from build123d import *

# Parameters (mm, degrees)
F3_DEPTH        = 4
F4_DEPTH        = 4
F7_D            = 3.2
F7_DEPTH        = 45
F7_TIP          = 0.9613769904
F8_D            = 28
F10_D           = 3.2
F10_DEPTH       = 60
F10_CSINK_D     = 6.72
F10_CSINK_ANGLE = 90
F10_TIP         = 0.9613769904
F12_DEPTH       = 4.0010001
F13_R           = 5


with BuildPart() as f3:
    # F0 (on Top) → F3 (new body)
    with BuildSketch(Plane.XY):
        with BuildLine():
            Line((-83.330666624, 34), (83.330666624, 34))
            ThreePointArc((83.330666624, 34), (73.1470337796, 52.4357840529), (58.9576118919, 68))
            Line((58.9576118919, 68), (-58.9576118919, 68))
            Line((-58.9576118919, 68), (-108.330666624, 68))
            Line((-108.330666624, 68), (-108.330666624, 34))
            Line((-108.330666624, 34), (-83.330666624, 34))
        make_face()
    extrude(amount=F3_DEPTH)

    # F0 (on Top) → F4 (join)
    with BuildSketch(Plane.XY):
        with BuildLine():
            Line((-83.330666624, 34), (83.330666624, 34))
            ThreePointArc((83.330666624, 34), (73.1470337796, 52.4357840529), (58.9576118919, 68))
            Line((58.9576118919, 68), (-58.9576118919, 68))
            Line((-58.9576118919, 68), (-108.330666624, 68))
            Line((-108.330666624, 68), (-108.330666624, 34))
            Line((-108.330666624, 34), (-83.330666624, 34))
        make_face()
    extrude(amount=F4_DEPTH)

    # F7
    with Locations(Plane.YZ.offset(83.3)):
        with Locations((63, 2), (39, 2)):
            Hole(F7_D / 2, depth=F7_DEPTH)
            with Locations((0, 0, -(F7_DEPTH + F7_TIP / 2))):  # 118° drill point
                Cone(0, F7_D / 2, F7_TIP, mode=Mode.SUBTRACT)

    # F8 (through all)
    with Locations(Plane(origin=(0, 0, 0), x_dir=(1, 0, 0), z_dir=(0, 0, -1))):
        with Locations((0, -52)):
            Hole(F8_D / 2)

    # F10
    with Locations(Plane.XY.offset(4)):
        with Locations((-103.330666624, 51), (-90.330666624, 51)):
            CounterSinkHole(F10_D / 2, F10_CSINK_D / 2, depth=F10_DEPTH, counter_sink_angle=F10_CSINK_ANGLE)
            with Locations((0, 0, -(F10_DEPTH + F10_TIP / 2))):  # 118° drill point
                Cone(0, F10_D / 2, F10_TIP, mode=Mode.SUBTRACT)

    # F11 (on face) → F12 (cut, through all)
    with BuildSketch(Plane.XY.offset(4)):
        with BuildLine():
            ThreePointArc((-81.8600177132, 38), (-73.8985762248, 51.8079427496), (-63.6322441848, 64))
            Line((-63.6322441848, 64), (-65.1300137514, 65.3254004397))
            ThreePointArc((-65.1300137514, 65.3254004397), (-75.5329519196, 52.9537515968), (-83.6166513022, 38.9561581637))
            Line((-83.6166513022, 38.9561581637), (-81.8600177132, 38))
        make_face()
    extrude(amount=-F12_DEPTH, mode=Mode.SUBTRACT)

    # F13
    f13_edges = [f3.edges().sort_by_distance(p)[0] for p in [
        (-108.330667, 34, 2),
        (-108.330667, 68, 2),
    ]]
    fillet(f13_edges, radius=F13_R)


solid = f3.part
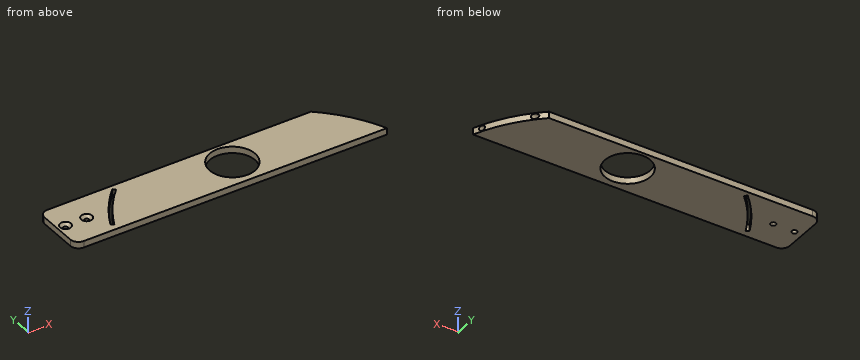
Geometry: final body of the model. Coordinates: model frame, mm. Round coordinates to 2 decimals unless told otherwise and drop trailing zeros. Loops run counter-clockwise (first coordinate to the right, second up) from the corner with the lowest first, then second, coordinate; pieces in that order, holes last. Notation, with made-up numbers: (80, 69) - (87, 69) arc R9 cw to (87, 73) - close; hole circle Ø1 at (33, -9.75). An arc over 180 degrees is marked (long way). Write each question's results on one line, items separated by ' | '. Start each with the question number.
1) Cut plane B-B on x = 48. Return loops of the section in (y, z), then the cut area to 3 significant figures.
2) Cut plane D-D on z = 1.2. Count the separate pieces of the cut face and the enclosed holes in it, then the cut area to 3 significant figures.
3) Cut plane C-C on y = 58. Return loops of the section in (x, z), then the cut area to 3 significant figures.
4) Cut plane A-A on x = 0. Return loops of the section in (y, z).
5) First-contact query: P1, Ø17, axis at x = 0, y = 52, coming from the -Z side. Flat tip, straight axial feed; report the tip coordinate or a pass-through.
6) Line query: probe 1 along Y at (x, z) = (46.75, 2); probe 2 along X at (y, z) = (42, 2.05); probe 3 along Y at (x, z) = (57, 3.25). Output: solid intervals per line, ascending. Write a range as [from, to].
Verdict:
1) outline: (34, 0) - (68, 0) - (68, 4) - (34, 4) - close; hole circle Ø3.2 at (39, 2); hole circle Ø3.2 at (63, 2) | area: 120 mm2
2) separate pieces: 1 | enclosed holes: 4 | area: 5,270 mm2
3) outline: (-108.33, 0) - (-71.73, 0) - (-71.73, 4) - (-108.33, 4) - close; (-69.15, 0) - (-12.65, 0) - (-12.65, 4) - (-69.15, 4) - close; (12.65, 0) - (68.82, 0) - (68.82, 4) - (12.65, 4) - close | area: 597 mm2
4) outline: (34, 0) - (38, 0) - (38, 4) - (34, 4) - close; (66, 0) - (68, 0) - (68, 4) - (66, 4) - close
5) P1: passes through
6) probe 1: y = [34, 37.4], [40.6, 61.4], [64.6, 68] | probe 2: x = [-108.33, -82.13], [-79.88, -9.8], [9.8, 79.6] | probe 3: y = [34, 38], [40, 62], [64, 68]
